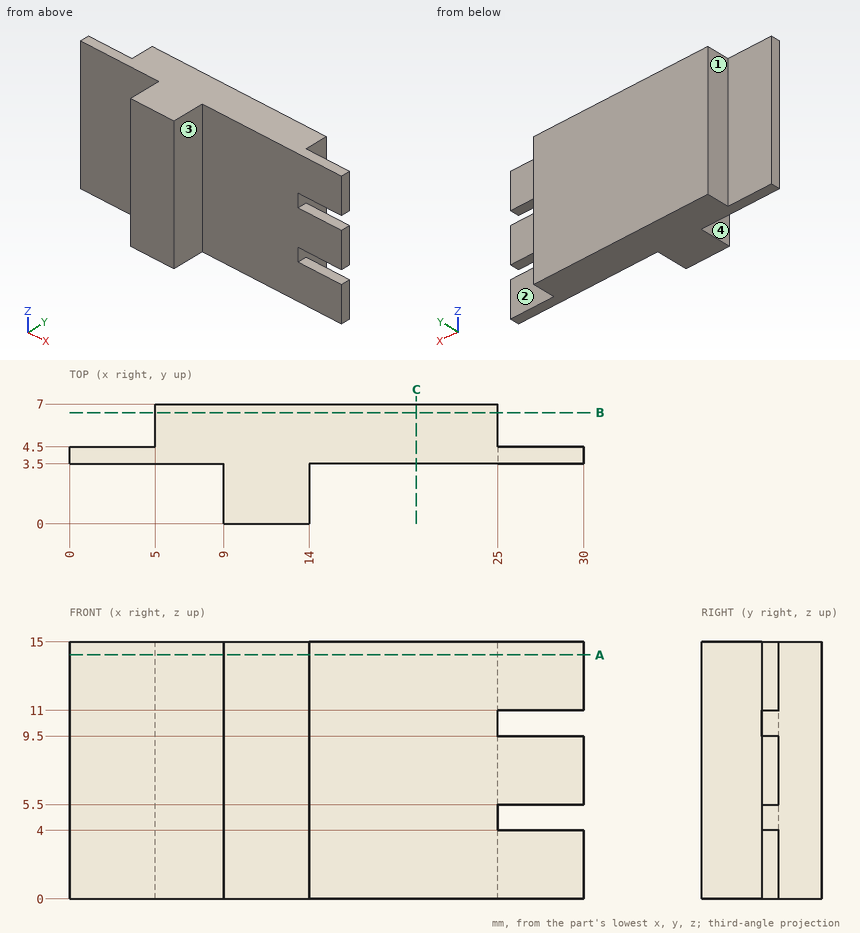
Here's the drawing with two shaded views (mm, measured from the low corner). I have some questions. A direction names the side the tool comes from. Coordinates: 2 decimals unless noted, no trailing zeros. Loops run counter-clockwise (first coordinate to the right, second up) from the corner with the lowest first, then second, coordinate; pieces in that order, holes last.
Item 1: Suppose I cut it at C-C (x = 20.25). Please give me the cut outline in (y, z), then the cut area to 3 significant figures.
Answers below:
outline: (3.5, 0) - (7, 0) - (7, 15) - (3.5, 15) - close
area: 52.5 mm2
Item 2: I'm going to push flat-ended pins straight in: pin 1 (1.5 mm diameter, centred on y = 2.5, z = 8, fed in from +X); pin 2 (1 mm diameter, centred on y = 1, z = 11, fed in from -X); pin 3 (2 mm diameter, centred on x = 28.5, z = 13.5, fed in from +Y). Where does each tip first touch, or does it pass through?
Answers below:
pin 1: stops at x = 14
pin 2: stops at x = 9
pin 3: stops at y = 4.5
Item 3: Suppose I cut it at B-B (y = 6.5). Please give me the cut outline in (x, z), then the cut area to 3 significant figures.
Answers below:
outline: (5, 0) - (25, 0) - (25, 15) - (5, 15) - close
area: 300 mm2
Item 4: Which directions (+Z, -Z, +X, -X, +Y, -Y) give clear straight access to the entire face, cutting with the end or side of a thin tool? Please do the marked faces 1, 2, 3 and 4.
Answers below:
face 1: +Z, -Z, -X, +Y
face 2: +Z, -Z, +X, +Y
face 3: +Z, -Z, +X, -Y
face 4: +Z, -Z, -X, -Y
Item 5: Suppose I cut it at A-A (z = 14.25). Please give me the cut outline in (x, y), then the cut area to 3 significant figures.
Answers below:
outline: (0, 3.5) - (9, 3.5) - (9, 0) - (14, 0) - (14, 3.5) - (30, 3.5) - (30, 4.5) - (25, 4.5) - (25, 7) - (5, 7) - (5, 4.5) - (0, 4.5) - close
area: 97.5 mm2
Item 6: Please list where these lines run through material, in increasing order: L1, parallel to Y at x = 14.5, z = 3.5; L2, parallel to X at y = 6.25, z = 8; L3, parallel to Y at x = 26.5, z = 12.
Answers below:
L1: y = 3.5 to 7
L2: x = 5 to 25
L3: y = 3.5 to 4.5
